Read the model definition and answer for the solid it produces. Units are mm, in the model's axes. Face numbers are marked on the shaded views. A direction names the side the tool comes from. Give positions to 0.01 mm unless a question says otherwise; leave off trailing zeros. Order: outer loops, then holes, each group sorted by start corner. A loop starts at its lowest first (then second) coordinate and runs counter-clockwise, first axis right, second up. Notation, with made-up numbers: (-18.5, 43.25) -> (-11.5, 43.25) arc R9 cw to (-11.5, 54.25) -> close; hole circle Ø10 at (69.25, 72.25). An arc over 180 degrees is marked (long way). Use one line per item in the form item = value.
```python
from build123d import *

# Parameters (mm, degrees)
BOSS_EXTRUDE1_DEPTH      = 12.7
BOSS_EXTRUDE1_DEPTH_BACK = 12.7
CUT_EXTRUDE1_DEPTH       = 27.549927447
CUT_EXTRUDE3_DEPTH       = 17.78
FILLET1_R                = 7.62
FILLET2_R                = 2.54


with BuildPart() as part:
    # Sketch1 → Boss-Extrude1 (new, two sides: drawn at the far end of the back side and taken through both)
    with BuildSketch(Plane(origin=(0, 0, 0), x_dir=(1, 0, 0), z_dir=(0, 1, 0)).offset(-BOSS_EXTRUDE1_DEPTH_BACK)):
        Polygon((-21.470544554, -2.672029703), (-8.770544554, -2.672029703), (-8.770544554, 19.552970297), (-11.945544554, 19.552970297), (-11.945544554, 0.502970297), (-18.295544554, 0.502970297), (-18.295544554, 19.552970297), (-21.470544554, 19.552970297), align=None)
    extrude(amount=BOSS_EXTRUDE1_DEPTH + BOSS_EXTRUDE1_DEPTH_BACK)

    # Sketch3 → Cut-Extrude1 (cut, through all)
    with BuildSketch(Plane.ZY.offset(21.470544554)):
        with BuildLine():
            ThreePointArc((-10.027970297, 3.175), (-13.202970297, 0), (-10.027970297, -3.175))
            Line((-10.027970297, -3.175), (-10.027970297, 0))
            Line((-10.027970297, 0), (-10.027970297, 3.175))
        make_face()
        with BuildLine():
            Line((-10.027970297, 0), (-10.027970297, -3.175))
            ThreePointArc((-10.027970297, -3.175), (-7.782906267, -2.24506403), (-6.852970297, 0))
            ThreePointArc((-6.852970297, 0), (-7.782906267, 2.24506403), (-10.027970297, 3.175))
            Line((-10.027970297, 3.175), (-10.027970297, 0))
        make_face()
    extrude(amount=-CUT_EXTRUDE1_DEPTH, mode=Mode.SUBTRACT)

    # Sketch5 → Cut-Extrude3 (cut)
    with BuildSketch(Plane(origin=(-8.770544554, 0, 0), x_dir=(0, 0, -1), z_dir=(1, 0, 0))):
        Polygon((19.552970297, 12.7), (9.369494421, 12.7), (19.552970297, 0), align=None)
        Polygon((19.552970297, -12.7), (19.552970297, 0), (9.369494421, -12.7), align=None)
    extrude(amount=-CUT_EXTRUDE3_DEPTH, mode=Mode.SUBTRACT)

    # Fillet1
    fillet1_edges = [part.edges().sort_by_distance(p)[0] for p in [
        (-19.883044554, 0, -19.552970297),
        (-10.358044554, 0, -19.552970297),
    ]]
    fillet(fillet1_edges, radius=FILLET1_R)

    # Fillet2
    fillet2_edges = [part.edges().sort_by_distance(p)[0] for p in [
        (-10.358044554, 12.7, -9.369494421),
        (-19.883044554, 12.7, -9.369494421),
        (-19.883044554, -12.7, -9.369494421),
        (-10.358044554, -12.7, -9.369494421),
    ]]
    fillet(fillet2_edges, radius=FILLET2_R)


solid = part.part
```
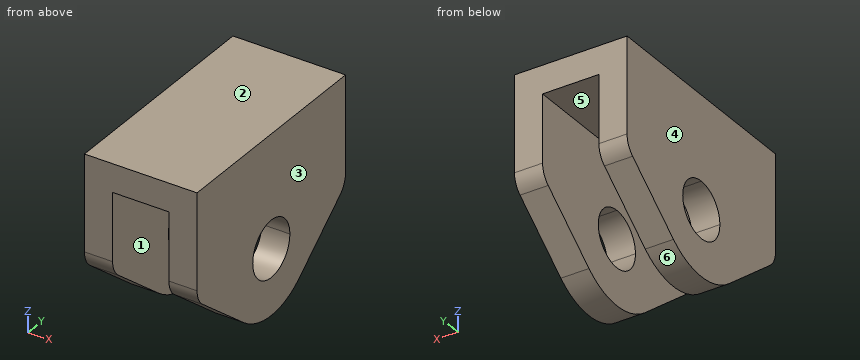
Item 1: The part is cut by section C-C on x = -10. Give the vertices of the cut face in (y, z) (3 decimals).
Checks:
outline = (-12.7, -8.15) arc R2.54 ccw to (-11.749, -10.132) -> (-4.767, -15.731) arc R7.62 ccw to (4.767, -15.731) -> (11.749, -10.132) arc R2.54 ccw to (12.7, -8.15) -> (12.7, 2.672) -> (-12.7, 2.672) -> close; hole circle Ø6.35 at (0, -10.028)
Item 2: Given pin 1 Ø4 at (x, z) = (-20, -12) entering from -Y; pin 2 Ø1.5 at (x, y) = (-13.5, 4) entering from -Z; pin 3 Ø4 at (x, z) = (-16, -13) entering from -Y, each flat-ended and moving along its own axis, determine where each tip first touches the part or whether it passes through.
Checks:
pin_1 = -11.9
pin_2 = -0.5
pin_3 = through
Item 3: The part is cut by section B-B on y = 2.75. Give the vertices of the cut face in (x, z), and give its area (3 significant figures).
Checks:
outline = (-21.47, -16.89) -> (-18.3, -16.89) -> (-18.3, -11.61) -> (-21.47, -11.61) -> close; (-21.47, -8.44) -> (-18.3, -8.44) -> (-18.3, -0.5) -> (-11.95, -0.5) -> (-11.95, -8.44) -> (-8.77, -8.44) -> (-8.77, 2.67) -> (-21.47, 2.67) -> close; (-11.95, -16.89) -> (-8.77, -16.89) -> (-8.77, -11.61) -> (-11.95, -11.61) -> close
area = 124 mm²
Item 4: Determine the mould class of the marked faces 3, 4, 5 and 6 for opening direction X: +X half, -X half, draft (parallel to the pull), parting line (faces both ways), or undercut.
Checks:
face_3 = +X half
face_4 = -X half
face_5 = undercut
face_6 = draft
Item 5: The part is cut by section A-A on z = -1.75. Give the vertices of the cut face in (x, y).
Checks:
outline = (-21.47, -12.7) -> (-18.3, -12.7) -> (-18.3, 12.7) -> (-21.47, 12.7) -> close; (-11.95, -12.7) -> (-8.77, -12.7) -> (-8.77, 12.7) -> (-11.95, 12.7) -> close
Item 6: Straight lines are drawn through the part: L1, parallel to X at y = 3.5, z = -3.25; L2, parallel to Z at x = -16.25, y = 3.5; L3, parallel to Y at x = -9.75, z = -9.25. For each, find the intervals that lie inside material, in ascending order. Write a range as from..to.
Checks:
L1 = -21.47..-18.3, -11.95..-8.77
L2 = -0.5..2.67
L3 = -12.45..-3.08, 3.08..12.45
Item 7: Which of the six approach directions +Z, -Z, +X, -X, +Y, -Y give full straight-line access (tool end or side, diameter ignored) to the marked faces 1 and 2?
Checks:
face_1 = -Z, +Y, -Y
face_2 = +Z, +X, -X, +Y, -Y
Item 8: The part is cut by section D-D on y = -3.75. Give the vertices of the cut face in (x, z).
Checks:
outline = (-21.47, -16.42) -> (-18.3, -16.42) -> (-18.3, -0.5) -> (-11.95, -0.5) -> (-11.95, -16.42) -> (-8.77, -16.42) -> (-8.77, 2.67) -> (-21.47, 2.67) -> close
